Here's how the part is built. I have some questions about the finished solid (model axes, mm). A direction names the side the tool comes from. Round coordinates to 2 decimals unless told otherwise and drop trailing zeros. Order: outer loops, then holes, each group sorted by start corner. A loop starts at its lowest first (then second) coordinate and runs counter-clockwise, first axis right, second up. Notation, with made-up numbers: (75.25, 25) -> (97.25, 25) arc R24 cw to (97.25, 59) -> close; hole circle Ø5 at (-18.75, 77). An arc over 180 degrees is marked (long way). Use a Markdown table: item, result. Add a question column.
from build123d import *

# Parameters (mm, degrees)
SKETCH009_W      = 4.24264
SKETCH009_H      = 4.24264
EXTRUDE004_DEPTH = 10


with BuildPart() as extrude004:
    # Sketch009 (on Face5 of Revolve001) → Extrude004 (new body)
    with BuildSketch(Plane.YZ.offset(30)):
        Rectangle(SKETCH009_W, SKETCH009_H)
    extrude(amount=-EXTRUDE004_DEPTH)


with BuildPart() as driven_wheel:
    # Sketch007 → Revolve001 (revolve)
    with BuildSketch(Plane.XZ):
        with BuildLine():
            Line((20, 4.5), (20, 0))
            Line((20, 0), (23.25, 0))
            Line((30, 0), (23.25, 0))
            Line((30, 12.875), (30, 0))
            ThreePointArc((30, 12.875), (29.816942, 13.316942), (29.375, 13.5))
            Line((28.125, 13.5), (29.375, 13.5))
            ThreePointArc((25.125, 13.5), (26.625, 12), (28.125, 13.5))
            Line((23.875, 13.5), (25.125, 13.5))
            ThreePointArc((23.875, 13.5), (23.433058, 13.316942), (23.25, 12.875))
            Line((23.25, 4.5), (23.25, 12.875))
            Line((23.25, 4.5), (20, 4.5))
        make_face()
    revolve(axis=Axis((0, 0, 0), (1, 0, 0)))

    # Cut: cut Extrude004
    add(extrude004.part, mode=Mode.SUBTRACT)


solid = driven_wheel.part
(1) I want a section at D-D on x = 25.75. List the corners of the cut face in (y, z) for me.
(2) I'm going to push flat-ended pins straight in: P1, Ø6, axis at x = 24, y = -6.5, coming from the -Z side; P2, Ø4, axis at x = 21.5, z = 8, coming from the +Y side; P3, Ø1.3, axis at x = 26.5, y = -0.5, coming from the +Z side. Where does each tip first touch, or does it pass through?
(3) If we mould it in two halves opening along Z, with no side actions, what happens to faces 4 (the flat face through (25, 0, -2.121)), 5 (the flat face through (20, 3, 0)), 6 (the cylindrical face through (24.51, 13.18, -2.93))? For each: pulls with the +Z half, pulls with the -Z half, needs draft (parallel to the pull), parting line crosses it, or undercut.
(4) I want a section at A-A on y = 0. List the corners of the cut face in (x, z) for me (3 decimals).
(5) Please list where these lines run through material, in increasing order: probe 1 along X at (y, z) = (2, -11); probe 2 along Y at (x, z) = (29.5, 0.25); probe 3 along Y at (x, z) = (23.5, 0.5). Write a range as from..to.
(6) I want a section at C-C on x = 21.75. List the corners of the cut face in (y, z) for me.
(7) On a 3-axis mill with a long thin cutter (end or side, diameter ignored), from which of +Z, -Z, +X, -X, +Y, -Y can I reach the whole of each face in a straight line? I mean faces 1 (the flat face through (23.25, 0, -6)), 2 (the flat face through (25, -2.121, 0)), 3 (the flat face through (30, 3, 0)). Say none if no direction works.
Output:
| question | item | result |
|---|---|---|
| 1 | outline | circle Ø24.56 at (0, 0); hole (-2.12, -2.12) -> (2.12, -2.12) -> (2.12, 2.12) -> (-2.12, 2.12) -> close |
| 2 | P1 | z = -13.04 |
| 2 | P2 | y = 11.06 |
| 2 | P3 | z = 12.21 |
| 3 | face 4 | undercut |
| 3 | face 5 | needs draft |
| 3 | face 6 | parting line crosses it |
| 4 | outline | (20, -4.5) -> (23.25, -4.5) -> (23.25, -12.875) arc R0.625 ccw to (23.875, -13.5) -> (25.125, -13.5) arc R1.5 cw to (28.125, -13.5) -> (29.375, -13.5) arc R0.625 ccw to (30, -12.875) -> (30, -2.121) -> (20, -2.121) -> close; (20, 2.121) -> (30, 2.121) -> (30, 12.875) arc R0.625 ccw to (29.375, 13.5) -> (28.125, 13.5) arc R1.5 cw to (25.125, 13.5) -> (23.875, 13.5) arc R0.625 ccw to (23.25, 12.875) -> (23.25, 4.5) -> (20, 4.5) -> close |
| 5 | probe 1 | 23.25..30 |
| 5 | probe 2 | -13.49..-2.12, 2.12..13.49 |
| 5 | probe 3 | -13.37..-2.12, 2.12..13.37 |
| 6 | outline | circle Ø9 at (0, 0); hole (-2.12, -2.12) -> (2.12, -2.12) -> (2.12, 2.12) -> (-2.12, 2.12) -> close |
| 7 | face 1 | -X |
| 7 | face 2 | +X, -X |
| 7 | face 3 | +Z, -Z, +X, +Y, -Y |
